from build123d import *

# Parameters (mm, degrees)
REVOLUTION_ANGLE     = -45
SKETCH001_W          = 200
SKETCH001_H          = 100
SKETCH001_W_2        = 40
SKETCH001_H_2        = 40
POCKET_DEPTH         = 146.825584
SKETCH002_R          = 2.15
POCKET001_DEPTH      = 20.001
POCKET001_DEPTH_BACK = -20.001
GROOVE_ANGLE         = -60
POCKET002_DEPTH      = 20.001
POCKET002_DEPTH_BACK = -20.001
POCKET003_DEPTH      = 4.001


with BuildPart() as part:
    # Sketch → Revolution (revolve, symmetric)
    with BuildSketch(Plane.XZ) as revolution_sk:
        with BuildLine():
            ThreePointArc((96.824584, -25), (100, 0), (96.824584, 25))
            Line((96.824584, 25), (146.824584, 25))
            Line((146.824584, 25), (146.824584, -25))
            Line((146.824584, -25), (96.824584, -25))
        make_face()
    revolve(axis=Axis((0, 0, 0), (0, 0, 1)), revolution_arc=REVOLUTION_ANGLE / 2)
    revolve(revolution_sk.sketch, axis=Axis((0, 0, 0), (0, 0, -1)), revolution_arc=REVOLUTION_ANGLE / 2)

    # Sketch001 → Pocket (cut, through all)
    with BuildSketch(Plane.YZ):
        Rectangle(SKETCH001_W, SKETCH001_H)
        Rectangle(SKETCH001_W_2, SKETCH001_H_2, mode=Mode.SUBTRACT)
    extrude(amount=POCKET_DEPTH, mode=Mode.SUBTRACT)

    # Sketch002 → Pocket001 (cut, two sides)
    with BuildSketch(Plane.XY) as pocket001_sk:
        with Locations((120, 0)):
            Circle(SKETCH002_R)
        with BuildLine():
            Line((120, 20), (120, 30))
            Line((120, 30), (150, 30))
            Line((150, 30), (150, -30))
            Line((150, -30), (120, -30))
            Line((120, -30), (120, -20))
            ThreePointArc((120, -20), (128.485281, -16.485281), (132, -8))
            Line((132, 8), (132, -8))
            ThreePointArc((132, 8), (128.485281, 16.485281), (120, 20))
        make_face()
    extrude(amount=-POCKET001_DEPTH, mode=Mode.SUBTRACT)
    extrude(pocket001_sk.sketch, amount=-POCKET001_DEPTH_BACK, mode=Mode.SUBTRACT)

    # Sketch003 → Groove (revolve, cut)
    with BuildSketch(Plane.XY.offset(-16)):
        with BuildLine():
            Line((159.136485, -18), (159.136485, 18))
            Line((159.136485, 18), (99.136485, 18))
            ThreePointArc((99.136485, -18), (100.737282, 0), (99.136485, 18))
            Line((99.136485, -18), (159.136485, -18))
        make_face()
    revolve(axis=Axis((0, 0, 0), (0, 1, 0)), revolution_arc=GROOVE_ANGLE, mode=Mode.SUBTRACT)

    # Sketch004 → Pocket002 (cut, two sides)
    with BuildSketch(Plane.XZ) as pocket002_sk:
        Polygon((102, 20.1), (124, -16), (154, -16), (154, 30.1), (102, 30.1), align=None)
    extrude(amount=-POCKET002_DEPTH, mode=Mode.SUBTRACT)
    extrude(pocket002_sk.sketch, amount=-POCKET002_DEPTH_BACK, mode=Mode.SUBTRACT)

    # Sketch005 → Pocket003 (cut, through all)
    with BuildSketch(Plane.XY.offset(-16)):
        with BuildLine():
            ThreePointArc((100.535935, -6.405797), (100.737282, 0), (100.535935, 6.405797))
            ThreePointArc((103.530013, 6.594203), (101.938771, 7.997039), (100.535935, 6.405797))
            ThreePointArc((103.530013, -6.594203), (103.737282, 0), (103.530013, 6.594203))
            ThreePointArc((100.535935, -6.405797), (101.938771, -7.997039), (103.530013, -6.594203))
        make_face()
    extrude(amount=-POCKET003_DEPTH, mode=Mode.SUBTRACT)


solid = part.part
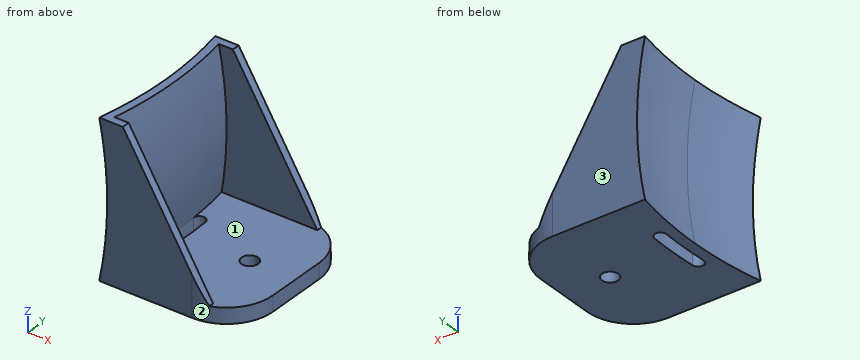
Could you check a few things on this model? Use its own coordinates, in mm. Face numbers are marked on the shaded views. Give positions to 0.01 mm unless a question says otherwise; leave off trailing zeros. Order: outer loops, then holes, each group sorted by start corner. A loop starts at its lowest first (then second) coordinate and runs counter-clockwise, first axis right, second up.
Item 1: I need wall thicknesses on line 1 (Y direction, x = 118, z = -9); line 2 (Y direction, x = 120, z = -17); line 3 (Z direction, x = 109, y = -7). Which ranges of each line are inside material? Lowest first, please.
Item 2: If we section it at C-C, the plane x = 107.5: Write out the boundary of the cut face in (y, z) (3 decimals).
Item 3: If we section it at A-A, the plane x = 121.5: Write out the boundary of the cut face in (y, z).
Item 4: I'm going to push flat-ended pins straight in: pin 1 (4 mm diameter, centred on y = -5.5, z = 7.5, fed in from -X); pin 2 (1.5 mm diameter, centred on y = -10, z = 10, fed in from -X); pin 3 (2 mm diameter, centred on y = -6.5, z = -5, fed in from -X). Where does each tip first touch, or does it pass through?
Item 5: If we section it at B-B, the plane x = 112.5: Write out the boundary of the cut face in (y, z).
Item 6: If we mould it in two halves opening along Y, with no side actions, what happens to the marked faces 1, 2 and 3? For each: pulls with the +Y half, pulls with the -Y half, needs draft (parallel to the pull), parting line crosses it, or undercut.
Values:
1. line 1: y = -20 to -18, 18 to 20
1. line 2: y = -20 to -2.15, 2.15 to 20
1. line 3: z = -20 to -16
2. outline: (-20, -20) - (20, -20) - (20, 11.075) - (18, 11.075) - (18, -16) - (-18, -16) - (-18, 11.075) - (-20, 11.075) - close
3. outline: (-19.91, -20) - (-1.54, -20) - (-1.54, -16) - (-18, -16) - (-18, -11.9) - (-19.91, -11.9) - close; (1.54, -20) - (19.91, -20) - (19.91, -11.9) - (18, -11.9) - (18, -16) - (1.54, -16) - close
4. pin 1: stops at x = 99.36
4. pin 2: stops at x = 98.88
4. pin 3: stops at x = 99.58
5. outline: (-20, -20) - (20, -20) - (20, 2.87) - (18, 2.87) - (18, -16) - (-18, -16) - (-18, 2.87) - (-20, 2.87) - close
6. face 1: undercut
6. face 2: pulls with the -Y half
6. face 3: pulls with the +Y half
